```python
from build123d import *

# Parameters (mm, degrees)
F1_DEPTH = 12.7
F3_DEPTH = 38.1
F4_R     = 5.08


# Not quite as in the source:
# - a feature of the source that left no trace in its solid (it failed there, or was rolled back) is left out


with BuildPart() as f1:
    # F0 (on Front) → F1 (new body, symmetric)
    with BuildSketch(Plane.XZ):
        with BuildLine():
            Line((-38.1, -38.1), (0, -38.1))
            Line((0, -38.1), (38.1, -38.1))
            ThreePointArc((38.1, -38.1), (43.6800141218, -27.583546173), (55.5166615897, -26.3083460258))
            Line((55.5166615897, -26.3083460258), (71.4833384103, 13.6083460258))
            ThreePointArc((71.4833384103, 13.6083460258), (63.7291538885, 27.8016655187), (76.2, 38.1))
            Line((76.2, 38.1), (0, 38.1))
            Line((0, 38.1), (-76.2, 38.1))
            ThreePointArc((-76.2, 38.1), (-67.2197438789, 34.3802561211), (-63.5, 25.4))
            ThreePointArc((-63.5, 25.4), (-65.683546173, 18.2800141218), (-71.4833384103, 13.6083460258))
            Line((-71.4833384103, 13.6083460258), (-55.5166615897, -26.3083460258))
            ThreePointArc((-55.5166615897, -26.3083460258), (-43.6800141218, -27.583546173), (-38.1, -38.1))
        make_face()
        with BuildLine():
            ThreePointArc((55.5166615897, -26.3083460258), (43.6800141218, -27.583546173), (38.1, -38.1))
            Line((38.1, -38.1), (44.45, -38.1))
            ThreePointArc((44.45, -38.1), (47.2400070609, -32.8417730865), (53.1583307948, -32.2041730129))
            Line((53.1583307948, -32.2041730129), (55.5166615897, -26.3083460258))
        make_face()
        with BuildLine():
            Line((-44.45, -38.1), (-38.1, -38.1))
            ThreePointArc((-38.1, -38.1), (-43.6800141218, -27.583546173), (-55.5166615897, -26.3083460258))
            Line((-55.5166615897, -26.3083460258), (-53.1583307948, -32.2041730129))
            ThreePointArc((-53.1583307948, -32.2041730129), (-47.2400070609, -32.8417730865), (-44.45, -38.1))
        make_face()
        with BuildLine():
            ThreePointArc((-76.2, 38.1), (-88.6708461115, 22.9983344813), (-71.4833384103, 13.6083460258))
            ThreePointArc((-71.4833384103, 13.6083460258), (-65.683546173, 18.2800141218), (-63.5, 25.4))
            ThreePointArc((-63.5, 25.4), (-67.2197438789, 34.3802561211), (-76.2, 38.1))
        make_face()
        with BuildLine():
            ThreePointArc((-69.85, 25.4), (-70.9417730865, 21.8400070609), (-73.8416692052, 19.5041730129))
            ThreePointArc((-73.8416692052, 19.5041730129), (-81.4582269135, 28.9599929391), (-69.85, 25.4))
        make_face(mode=Mode.SUBTRACT)
        with BuildLine():
            ThreePointArc((76.2, 38.1), (63.7291538885, 27.8016655187), (71.4833384103, 13.6083460258))
            ThreePointArc((71.4833384103, 13.6083460258), (83.3199858782, 14.883546173), (88.9, 25.4))
            ThreePointArc((88.9, 25.4), (85.1802561211, 34.3802561211), (76.2, 38.1))
        make_face()
        with BuildLine():
            ThreePointArc((82.55, 25.4), (79.7599929391, 20.1417730865), (73.8416692052, 19.5041730129))
            ThreePointArc((73.8416692052, 19.5041730129), (72.6400070609, 30.6582269135), (82.55, 25.4))
        make_face(mode=Mode.SUBTRACT)
        with BuildLine():
            ThreePointArc((-55.5166615897, -26.3083460258), (-57.9199858782, -48.616453827), (-38.1, -38.1))
            Line((-38.1, -38.1), (-44.45, -38.1))
            ThreePointArc((-44.45, -38.1), (-54.3599929391, -43.3582269135), (-53.1583307948, -32.2041730129))
            Line((-53.1583307948, -32.2041730129), (-55.5166615897, -26.3083460258))
        make_face()
        with BuildLine():
            Line((44.45, -38.1), (38.1, -38.1))
            ThreePointArc((38.1, -38.1), (50.8, -50.8), (63.5, -38.1))
            ThreePointArc((63.5, -38.1), (61.316453827, -30.9800141218), (55.5166615897, -26.3083460258))
            Line((55.5166615897, -26.3083460258), (53.1583307948, -32.2041730129))
            ThreePointArc((53.1583307948, -32.2041730129), (56.0582269135, -34.5400070609), (57.15, -38.1))
            ThreePointArc((57.15, -38.1), (50.8, -44.45), (44.45, -38.1))
        make_face()
    extrude(amount=F1_DEPTH, both=True)

    # F2 (on Front) → F3 (cut)
    with BuildSketch(Plane.XZ):
        Polygon((-38.1, -19.05), (0, -19.05), (38.1, -19.05), (58.42, 38.1), (0, 38.1), (-58.42, 38.1), align=None)
    extrude(amount=F3_DEPTH, mode=Mode.SUBTRACT)

    # F4
    f4_edges = [f1.edges().sort_by_distance(p)[0] for p in [
        (-38.1, -6.35, -19.05),
        (38.1, -6.35, -19.05),
    ]]
    fillet(f4_edges, radius=F4_R)


solid = f1.part
```
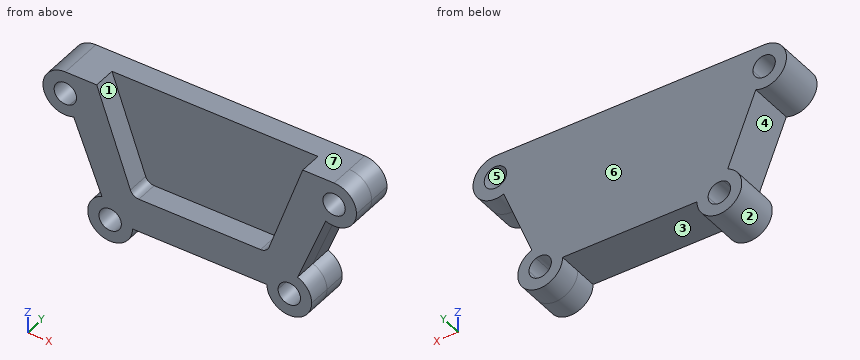
Can you work these out from the model? Positions are in its coordinate system, mm. Face numbers are marked on the shaded views. A direction names the side the tool comes from. Coordinates: 2 decimals unless noted, no trailing zeros. Order: outer loops, then holes, each group sorted by start corner. A loop starts at its lowest first (then second) coordinate and runs counter-clockwise, first axis right, second up.
1. I need wall thicknesses on line 1 (X direction, y = 3.75, z = 25.4); line 2 (Z direction, x = -76.2, y = 2.5); line 3 (X direction, y = -1.5, z = 25). Which ranges of each line are inside material? Lowest first, please.
2. If we section it at A-A (y = -8.5): Please give me the cut outline in (x, z), then the cut area to 3 significant figures.
3. For the marked faces 1, 2 and 3, which set-ups out of +Z, -Z, +X, -X, +Y, -Y let a thin tool reach every point of the face, with its end or its side?
4. If we section it at D-D (z = -6): Please give me the cut outline in (x, y), then the cut area to 3 significant figures.
5. If we section it at C-C (z = 23.5): Please give me the cut outline in (x, y).
6. Thinking about a two-plate mould opening in Z: for the marked faces 4, 5, 6 and 7, which applies, +Z half, -Z half, draft (parallel to the pull), parting line (faces both ways), or undercut?
7. If we section it at B-B (x = -50.8): Please give me the cut outline in (y, z).
8. I'm going to push flat-ended pins straight in: pin 1 (1.5 mm diameter, centred on y = 1.5, z = -9, fed in from +X); pin 2 (4 mm diameter, centred on x = -16, y = -5, fed in from +Z); pin 3 (5 mm diameter, centred on y = 4, z = -24.5, fed in from +X). Where does each tip first touch, or does it pass through?
Entries:
1. line 1: x = -88.9 to -82.55, -69.85 to 69.85, 82.55 to 88.9
1. line 2: z = 12.7 to 19.05, 31.75 to 38.1
1. line 3: x = -88.89 to -82.54, -69.86 to -53.76, 53.76 to 69.86, 82.54 to 88.89
2. outline: (-76.2, 38.1) arc R12.7 ccw (long way) to (-71.48, 13.61) - (-55.52, -26.31) arc R12.7 ccw (long way) to (-38.1, -38.1) - (38.1, -38.1) arc R12.7 ccw (long way) to (55.52, -26.31) - (71.48, 13.61) arc R12.7 ccw (long way) to (76.2, 38.1) - (58.42, 38.1) - (39.3, -15.67) arc R5.08 cw to (34.51, -19.05) - (-34.51, -19.05) arc R5.08 cw to (-39.3, -15.67) - (-58.42, 38.1) - close; hole circle Ø12.7 at (-76.2, 25.4); hole circle Ø12.7 at (-50.8, -38.1); hole circle Ø12.7 at (50.8, -38.1); hole circle Ø12.7 at (76.2, 25.4)
2. area: 5,250 mm2
3. face 1: +Z, -Y
3. face 2: +Y, -Y
3. face 3: -Z, +Y, -Y
4. outline: (-63.64, -12.7) - (-42.74, -12.7) - (-42.74, 0) - (42.74, 0) - (42.74, -12.7) - (63.64, -12.7) - (63.64, 12.7) - (-63.64, 12.7) - close
4. area: 2,150 mm2
5. outline: (-88.76, -12.7) - (-82.26, -12.7) - (-82.26, 12.7) - (-88.76, 12.7) - close; (-70.14, -12.7) - (-53.23, -12.7) - (-53.23, 0) - (53.23, 0) - (53.23, -12.7) - (70.14, -12.7) - (70.14, 12.7) - (-70.14, 12.7) - close; (82.26, -12.7) - (88.76, -12.7) - (88.76, 12.7) - (82.26, 12.7) - close
6. face 4: undercut
6. face 5: undercut
6. face 6: draft
6. face 7: +Z half
7. outline: (-12.7, -50.8) - (12.7, -50.8) - (12.7, -44.45) - (-12.7, -44.45) - close; (-12.7, -31.75) - (12.7, -31.75) - (12.7, 38.1) - (0, 38.1) - (0, 16.67) - (-12.7, 16.67) - close
8. pin 1: stops at x = 62.74
8. pin 2: stops at z = -19.05
8. pin 3: stops at x = 57.24
